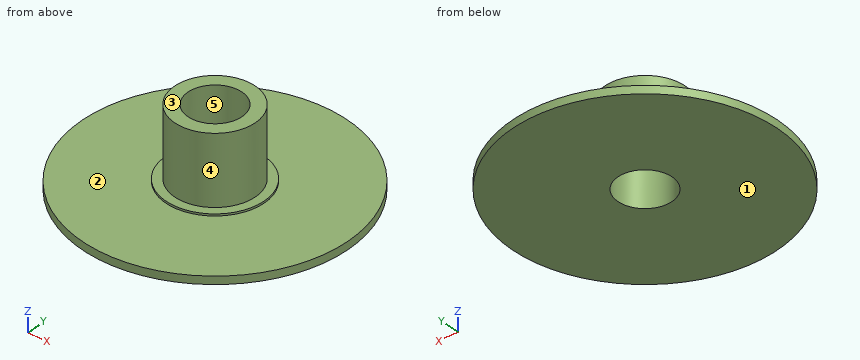
```python
from build123d import *

# Parameters (mm, degrees)
F0_R     = 13.5
F0_R_2   = 5
F1_DEPTH = 0.8
F0_R_3   = 4.1
F0_R_4   = 2.75
F2_DEPTH = 8
F3_DEPTH = 1


with BuildPart() as f1:
    # F0 (on Top) → F1 (new body)
    with BuildSketch(Plane.XY):
        Circle(F0_R)
        Circle(F0_R_2, mode=Mode.SUBTRACT)
    extrude(amount=F1_DEPTH)



with BuildPart() as f2:
    # F0 (on Top) → F2 (new body)
    with BuildSketch(Plane.XY):
        Circle(F0_R_3)
        Circle(F0_R_4, mode=Mode.SUBTRACT)
    extrude(amount=F2_DEPTH)


with BuildPart() as f1_1:
    add(f1.part)

    add(f2.part)  # F3 merges F2
    # F0 (on Top) → F3 (join)
    with BuildSketch(Plane.XY):
        Circle(F0_R_2)
        Circle(F0_R_3, mode=Mode.SUBTRACT)
    extrude(amount=F3_DEPTH)


solid = f1_1.part
```
Part model, mm, in its own coordinate system. Face numbers are marked on the shaded views. A direction names the side the tool comes from. Round coordinates to 2 decimals unless told otherwise and drop trailing zeros. Write each loop counter-clockwise with the first axis right and the second up, starting at its lowest first coordinate (ties: lowest second). Pieces come first, ordered by that corner, then holes. Notation, with made-up numbers: M 45.25,6.25 L 100.25,6.25 A9 cw 100.25,11.25 Z; hole C -33.5,75.5 d5. An arc over 180 degrees is marked long. One line per question, with ' | ' between items.
(1) Probe line 1 along Y through (x, z) = (0, 6.5); line 2 along Z through (x, y) = (-4.5, -3.75); line 3 along Y through (x, z) = (1.5, 7.5). List the from-to ranges inside material, lowest first.
Answer key:
line 1: y = -4.1 to -2.75, 2.75 to 4.1 | line 2: z = 0 to 0.8 | line 3: y = -3.82 to -2.3, 2.3 to 3.82
(2) Saw through at A-A on y = 0. Write the cut outline in (x, z), then the cut area to 3 significant figures.
Answer key:
outline: M -13.5,0 L -2.75,0 L -2.75,8 L -4.1,8 L -4.1,1 L -5,1 L -5,0.8 L -13.5,0.8 Z; M 2.75,0 L 13.5,0 L 13.5,0.8 L 5,0.8 L 5,1 L 4.1,1 L 4.1,8 L 2.75,8 Z | area: 37.0 mm^2
(3) Saw through at D-D on y = 3.5. Write the cut outline in (x, z), then the cut area to 3 significant figures.
Answer key:
outline: M -13.04,0 L 13.04,0 L 13.04,0.8 L 3.57,0.8 L 3.57,1 L 2.14,1 L 2.14,8 L -2.14,8 L -2.14,1 L -3.57,1 L -3.57,0.8 L -13.04,0.8 Z | area: 52.2 mm^2
(4) Two-plate mould, pull along Y, no slides. Class the marked faces 3, 4 and 5: released by +Y, released by -Y, zero draft, split by the parting line, or undercut.
Answer key:
face 3: zero draft | face 4: split by the parting line | face 5: undercut
(5) Saw through at C-C on z = 6.5. Write the cut outline in (x, y), then the cut area to 3 significant figures.
Answer key:
outline: C 0,0 d8.2; hole C 0,0 d5.5 | area: 29.1 mm^2
(6) Pin check, flat tips, straight feed: pin 1 (2 mm diameter, centred on x = 4, z = 4, fed in from -Y); pin 2 (4 mm diameter, centred on y = 9.5, z = 1, fed in from -X); pin 3 (1.5 mm diameter, centred on y = 0.5, z = 5.5, fed in from +X). Stop position of each tip, or through.
Answer key:
pin 1: stops at y = -2.79 | pin 2: stops at x = -11.22 | pin 3: stops at x = 4.1
(7) 3-axis set-ups, long thin cutter, end or side, ignore diameter. For the marked faces 1 and 2: which of +Z, -Z, +X, -X, +Y, -Y reach the whole face in a straight line?
Answer key:
face 1: -Z, +X, -X, +Y, -Y | face 2: +Z
